Autodesk Inventor part; units mm, degrees
ref_plane "YZ Plane" through (0, 0, 0) normal (1, 0, 0) x (0, 1, 0)
ref_plane "XZ Plane" through (0, 0, 0) normal (0, 1, 0) x (-1, 0, 0)
ref_plane "XY Plane" through (0, 0, 0) normal (0, 0, 1) x (1, 0, 0)
sketch "Sketch1" plane through (0, 0, 0) normal (0, 1, 0) x (-1, 0, 0)
  line L0 (-13, -5) -> (13, -5)
  line L1 (13, -5) -> (13, 5)
  line L2 (13, 5) -> (-13, 5)
  line L3 (-13, 5) -> (-13, -5)
  line L4 (-13, -5) -> (13, 5) construction
  line L5 (13, -5) -> (-13, 5) construction
  point P0 (0, 0)
  dimension "d0" = 26
  dimension "d1" = 10
extrude "Extrusion1" add sketch "Sketch1" along normal blind 14
sketch "Sketch2" plane through (0, 0, 0) normal (0, -1, 0) x (1, 0, 0)
  line L0 (13, -5) -> (-13, -5)
  line L1 (13, 5) -> (13, -5)
  line L2 (-13, 5) -> (13, 5)
  line L3 (-13, -5) -> (-13, 5)
  line L4 (-4.5, 3) -> (4.5, 3)
  line L5 (4.5, 3) -> (4.5, -5)
  line L6 (4.5, -5) -> (-4.5, -5)
  line L7 (-4.5, -5) -> (-4.5, 3)
  line L8 (-4.5, 3) -> (4.5, -5) construction
  line L9 (4.5, 3) -> (-4.5, -5) construction
  point P0 (0, 0)
  point P1 (0, -1)
  dimension "d4" = 9
  dimension "d5" = 4.5
  dimension "d6" = 8
extrude "Extrusion2" cut sketch "Sketch2" against normal blind 3 contours L0 L7 L4 L5
fillet "Fillet1" radius 3 2 edges at (-4.5, 1.5, -5) (4.5, 1.5, -5)
sketch "Sketch3" plane through (0, 3, 0) normal (0, -1, 0) x (1, 0, 0)
  line L0 (-4.5, 3) -> (4.5, 3)
  point P0 (0, 0)
  point P1 (0, -1.1)
  dimension "d10" = 4.1
hole "Hole1" at (0, 3, -1.1) direction (0, 1, 0) diameter 4 end through all
sketch "Sketch4" plane through (13, 14, -5) normal (0, 0, -1) x (-1, 0, 0)
  line L0 (5.5, -11) -> (20.5, -11)
  line L1 (20.5, -14) -> (20.5, -11)
  line L2 (20.5, -14) -> (26, -14)
  line L3 (26, -14) -> (26, 0)
  line L4 (0, 0) -> (26, 0)
  line L5 (0, -14) -> (0, 0)
  line L6 (0, -14) -> (5.5, -14)
  line L7 (5.5, -11) -> (5.5, -14)
  line L8 (0, -14) -> (0, 0)
  line L9 (0, -14) -> (1, -14)
  line L10 (1, -14) -> (1, 0)
  line L11 (1, 0) -> (0, 0)
  line L12 (0, 0) -> (0, -14)
  line L13 (20.5, -14) -> (26, -14)
  line L14 (26, -14) -> (25, -14)
  line L15 (25, -14) -> (25, 0)
  line L16 (25, 0) -> (26, 0)
  line L17 (26, 0) -> (26, -14)
  line L18 (1, -2) -> (25, -2)
  line L19 (25, -2) -> (25, 0)
  line L20 (25, 0) -> (1, 0)
  line L21 (1, 0) -> (1, -2)
  point P0 (13, -14)
  dimension "d18" = 1
  dimension "d19" = 1
  dimension "d20" = 2
extrude "Extrusion3" add sketch "Sketch4" along normal blind 35 contours L6 L5 L4 L10 | L15 L4 L3 L2 | L10 L4 L15 L18
sketch "Sketch5" plane through (0, 14, 0) normal (0, 1, 0) x (1, 0, 0)
  circle A0 centre (0, 1.1) radius 2
  circle A1 centre (0, 1.1) radius 3
  point P0 (0, 0)
  dimension "d23" = 6
extrude "Extrusion4" cut sketch "Sketch5" against normal blind 2
fillet "Fillet2" radius 8 1 edges at (0, 14, 5)
sketch "Sketch6" plane through (0, 0, 0) normal (0, -1, 0) x (1, 0, 0)
  arc A0 (4.5, -2) -> (7.5, -5) centre (7.5, -2) ccw
  line L0 (12, -5) -> (7.5, -5)
  line L1 (12, -5) -> (12, -40)
  line L2 (13, -40) -> (12, -40)
  line L3 (13, 5) -> (13, -40)
  line L4 (-13, 5) -> (13, 5)
  line L5 (-13, 5) -> (-13, -40)
  line L6 (-12, -40) -> (-13, -40)
  line L7 (-12, -5) -> (-12, -40)
  line L8 (-7.5, -5) -> (-12, -5)
  arc A1 (-7.5, -5) -> (-4.5, -2) centre (-7.5, -2) ccw
  line L9 (-4.5, -2) -> (-4.5, 3)
  line L10 (-4.5, 3) -> (4.5, 3)
  line L11 (4.5, 3) -> (4.5, -2)
  point P0 (0, 0)
extrude "Extrusion5" add sketch "Sketch6" along normal blind 10
fillet "Fillet3" radius 3 2 edges at (12, 12, -22.5) (-12, 12, -22.5)
fillet "Fillet4" radius 3 6 edges at (13, 11.6569, 2.6569) (13, -2, 5) (13, 14, -21.5) (-13, 11.6569, 2.6569) (-13, -2, 5) (-13, 14, -21.5)
sketch "Sketch7" plane through (0, -10, 0) normal (0, -1, 0) x (1, 0, 0)
  point P0 (0, 0)
sketch "Sketch8" plane through (0, -10, 0) normal (0, -1, 0) x (1, 0, 0)
  line L0 (9.9543, -5) -> (-10.0457, -5)
  line L1 (-10.0457, -5) -> (-10.0457, 4.3303)
  line L2 (-10.0457, 4.3303) -> (9.9543, 4.3303)
  line L3 (9.9543, 4.3303) -> (9.9543, -5)
  line L4 (7.5, -5) -> (-7.5, -5)
  point P0 (0, 0)
  dimension "d33" = 20
  dimension "d34" = 0
extrude "Extrusion6" add sketch "Sketch8" against normal blind 9.5
sketch "Sketch9" plane through (0, 3, 0) normal (0, -1, 0) x (1, 0, 0)
  circle A0 centre (0, -1.1) radius 2
  point P0 (0, 0)
extrude "Extrusion7" cut sketch "Sketch9" along normal through all
properties part number "little_rays_shell"
For this review, take the finished solid that the model builds, in its own axes (mm). A direction names the side the tool comes from. Round coordinates to 2 decimals unless told otherwise and drop trailing zeros. Write each loop counter-clockwise with the first axis right and the second up, starting at its lowest first coordinate (ties: lowest second). Pieces come first, ordered by that corner, then holes. Notation, with made-up numbers: (-2.75, -1) - (9.25, -1) arc R35 cw to (9.25, 36) - close; hole circle Ø10 at (89, 54). An arc over 180 degrees is marked (long way). Use a Markdown table: item, result.
Q1. We need section C-C (x = 3.75). Give the boundary of the cut face in (y, z), plus the area to 3 significant figures.
Derived:
| item | result |
|---|---|
| outline | (-10, -5) - (-0.5, -5) - (-0.5, 3) - (3, 3) - (3, -5) - (12, -5) - (12, -40) - (14, -40) - (14, -3) arc R8 ccw to (6, 5) - (-10, 5) - close |
| area | 268 mm2 |
Q2. The part is to be moulded in two halves that separate along Z. For faces 1 (the cylindrical face through (5.4, 1.27, -4.14)), 2 (the cylindrical face through (-0.14, 11.594, 2.719)), 3 (the flat face through (1, -10, -4)), 4 (the cylindrical face through (-0.26, -5.183, -3.083)), say which applies: pulls with the +Z half, pulls with the -Z half, needs draft (parallel to the pull), parting line crosses it, or undercut.
Derived:
| item | result |
|---|---|
| face 1 | pulls with the -Z half |
| face 2 | pulls with the +Z half |
| face 3 | needs draft |
| face 4 | undercut |
Q3. We need section A-A (y = 1.25). Give the boundary of the cut face in (x, z), plus the area to 3 significant figures.
Derived:
| item | result |
|---|---|
| outline | (-13, -40) - (-12, -40) - (-12, -5) - (-7.5, -5) arc R3 ccw to (-4.5, -2) - (-4.5, 3) - (4.5, 3) - (4.5, -2) arc R3 ccw to (7.5, -5) - (12, -5) - (12, -40) - (13, -40) - (13, 2) arc R3 ccw to (10, 5) - (-10, 5) arc R3 ccw to (-13, 2) - close |
| area | 250 mm2 |
Q4. We need section D-D (y = 4.5). Give the boundary of the cut face in (x, z).
Derived:
| item | result |
|---|---|
| outline | (-13, -40) - (-12, -40) - (-12, -5) - (12, -5) - (12, -40) - (13, -40) - (13, 2) arc R3 ccw to (10, 5) - (-10, 5) arc R3 ccw to (-13, 2) - close; hole circle Ø4 at (0, -1.1) |
Q5. We need section B-B (z = -14.5). Give the boundary of the cut face in (x, y), plus the area to 3 significant figures.
Derived:
| item | result |
|---|---|
| outline | (-13, -10) - (-12, -10) - (-12, 9) arc R3 cw to (-9, 12) - (9, 12) arc R3 cw to (12, 9) - (12, -10) - (13, -10) - (13, 11) arc R3 ccw to (10, 14) - (-10, 14) arc R3 ccw to (-13, 11) - close |
| area | 96.0 mm2 |
Q6. Machinability: for faces 5 (the flat face through (4.5, 1, 1)), 6 (the cylindrical face through (-12.14, -1.89, 4.1)), 7 (the cylindrical face through (-11.14, 11.1, -22.74)), 8 (the flat face through (1, 12, 1)), which of the approach directions +Z, -Z, +X, -X, +Y, -Y give a long, thin tool a straight path to every point of the face, cutting with its end or side? Answer none if there is none.
Derived:
| item | result |
|---|---|
| face 5 | -Z |
| face 6 | +Z, -X, +Y, -Y |
| face 7 | -Z, -Y |
| face 8 | +Y |
Q7. Clearance check with flat-ended pins moving along their axes: pin 1 (6.5 mm diameter, centred on x = -0.5, z = 0, fed in from +Y); pin 2 (1.5 mm diameter, centred on x = 3.5, y = 1, fed in from -Z); pin 3 (4 mm diameter, centred on x = -8.5, z = -13, fed in from -Y). State where each tip first meets the part, or that it passes through.
Derived:
| item | result |
|---|---|
| pin 1 | stops at y = 13.98 |
| pin 2 | stops at z = 3 |
| pin 3 | stops at y = 11.6 |
Q8. Wall thickness on line 1 along X through (y, z) = (-7.25, -1.1); line 2 along X through (y, z) = (7, -26.5); line 3 along Z through (x, y) = (0, -3): over which ranges is each line inside the solid? List them lowest first.
Derived:
| item | result |
|---|---|
| line 1 | x = -13 to -2, 2 to 13 |
| line 2 | x = -13 to -12, 12 to 13 |
| line 3 | z = -5 to -3.1, 0.9 to 5 |
